Source: CAD feature listing. Evaluate the final solid. Frame: model axes, mm. A direction names the side the tool comes from. Give positions to 0.01 mm unless a question says otherwise; leave off trailing zeros. Order: outer loops, then holes, each group sorted by start corner. A loop starts at its lowest first (then second) coordinate and runs counter-clockwise, first axis right, second up. Notation, with made-up numbers: (3.25, -7) - (43.25, -7) arc R35 cw to (43.25, 29) - close; hole circle Ø9 at (54, -30). An arc over 180 degrees is marked (long way). Write each question's results on one line, items separated by ' | '. Start each with the question number.
Item 1: Line query: line 1 along Y through (x, z) = (0, 20); line 2 along X through (y, z) = (-5.5, 19); line 3 along Y through (x, z) = (2.5, 26). Output: solid intervals per line, ascending.
Item 2: Set-up query: faces 4 (the cylindrical face through (-0.04, -23.31, 21.84)), 5 (the flat face through (15, 15, 4)), 6 (the flat face through (2.5, -19, 20)), 7 (the flat face through (0, -19, 15)), 8 (the cylindrical face through (23.773, 23.602, 38.028)). Return all of +Z, -Z, +X, -X, +Y, -Y with unobstructed straight access to the full face (end or side cutting, diameter ignored); none if empty.
Item 3: Section D-D on z = 34. Output: boundary loops of the cut face in (x, y).
Item 4: Contact query for flat-ended pins moving along their axis: pin 1 Ø1 at (x, y) = (1.5, -16) entering from +Z; pin 2 Ø2 at (x, z) = (6, 19.5) entering from -Y; pin 3 Ø5 at (y, z) = (-24.5, 19) entering from -X. Output: stop coordinate, or through.
Item 5: Section C-C on x = 14.5. Output: boundary loops of the cut face in (y, z).
Item 6: Mould query, pull axis Z, two halves, no side actions, for faces 1 (the flat face through (0, -19, 25)), 2 (the flat face through (15, 15, 36)), 3 (the flat face through (-2.5, -19, 20)). Classes: released by +Z, released by -Z, zero draft, split by the parting line, or undercut.
Item 7: Section A-A on z = 20. Output: boundary loops of the cut face in (x, y), and give its area (3 significant figures).
Item 8: Section B-B on y = -1. Output: boundary loops of the cut face in (x, z).
```python
from build123d import *

# Parameters (mm, degrees)
EXTRUDE_1_DEPTH      = 40
SKETCH_1_4_R         = 3
EXTRUDE_3_DEPTH      = 4
EXTRUDE_4_DEPTH      = 2.5
EXTRUDE_4_DEPTH_BACK = 2.5
SKETCH_2_R           = 2.5


with BuildPart() as part:
    # Sketch 1 → Extrude 1 (new body)
    with BuildSketch(Plane.XY):
        with BuildLine():
            ThreePointArc((7.494638572, -0.283536021), (-5.303300859, -5.303300859), (-0.283536021, 7.494638572))
            Line((-0.283536021, 7.494638572), (4.048166637, 11.82634123))
            ThreePointArc((4.048166637, 11.82634123), (-10.169859462, -7.268009254), (12.5, 0))
            ThreePointArc((12.5, 0), (12.330435219, 2.05191796), (11.82634123, 4.048166637))
            Line((11.82634123, 4.048166637), (7.494638572, -0.283536021))
        make_face()
        with BuildLine():
            Line((4.048166637, 11.82634123), (-0.283536021, 7.494638572))
            ThreePointArc((-0.283536021, 7.494638572), (5.202089957, 5.40261604), (7.5, 0))
            ThreePointArc((7.5, 0), (7.498659523, -0.141793353), (7.494638572, -0.283536021))
            Line((7.494638572, -0.283536021), (11.82634123, 4.048166637))
            ThreePointArc((11.82634123, 4.048166637), (8.838834765, 8.838834765), (4.048166637, 11.82634123))
        make_face()
    extrude(amount=EXTRUDE_1_DEPTH)

    # Sketch 1_4 → Extrude 3 (add)
    with BuildSketch(Plane.XY):
        with BuildLine():
            Line((15.909902577, 23.68807717), (4.048166637, 11.82634123))
            ThreePointArc((4.048166637, 11.82634123), (8.838834765, 8.838834765), (11.82634123, 4.048166637))
            Line((11.82634123, 4.048166637), (23.68807717, 15.909902577))
            ThreePointArc((23.68807717, 15.909902577), (23.68807717, 23.68807717), (15.909902577, 23.68807717))
        make_face()
        with Locations((19.798989873, 19.798989873)):
            Circle(SKETCH_1_4_R, mode=Mode.SUBTRACT)
    extrude_3 = extrude(amount=EXTRUDE_3_DEPTH)

    # Mirror 1: Extrude 3 across plane
    add(extrude_3.mirror(Plane.XY.offset(20)))

    # Sketch 2 → Extrude 4 (add, two sides: drawn at the far end of the back side and taken through both)
    with BuildSketch(Plane(origin=(0, 0, 0), x_dir=(0, 0, -1), z_dir=(1, 0, 0)).offset(-EXTRUDE_4_DEPTH_BACK)):
        with BuildLine():
            Line((-25, -12.5), (-25, -25))
            ThreePointArc((-25, -25), (-20, -30), (-15, -25))
            Line((-15, -25), (-15, -12.5))
            ThreePointArc((-15, -12.5), (-15.105468435, -11.478451782), (-15.417424305, -10.5))
            Line((-15.417424305, -10.5), (-24.582575695, -10.5))
            ThreePointArc((-24.582575695, -10.5), (-24.894531565, -11.478451782), (-25, -12.5))
        make_face()
        with Locations((-20, -25)):
            Circle(SKETCH_2_R, mode=Mode.SUBTRACT)
    extrude(amount=EXTRUDE_4_DEPTH + EXTRUDE_4_DEPTH_BACK)


solid = part.part
```
Evaluation:
1) line 1: y = -30 to -27.5, -22.5 to -7.5, 7.5 to 12.5 | line 2: x = -11.22 to -5.1, 5.1 to 11.22 | line 3: y = -12.25 to -7.07, 7.07 to 12.25
2) face 4: +X, -X | face 5: +X, +Y | face 6: +Z, -Z, +X, -Y | face 7: -Z, +X, -X, -Y | face 8: +Z, -Z
3) outline: circle Ø25 at (0, 0); hole (7.49, -0.28) arc R7.5 ccw to (7.5, 0) arc R7.5 ccw (long way) to start
4) pin 1: stops at z = 25 | pin 2: stops at y = -11.46 | pin 3: stops at x = -2.5
5) outline: (6.72, 0) - (22.28, 0) - (22.28, 4) - (6.72, 4) - close; (6.72, 36) - (22.28, 36) - (22.28, 40) - (6.72, 40) - close
6) face 1: released by +Z | face 2: undercut | face 3: zero draft
7) outline: (-2.5, -30) - (2.5, -30) - (2.5, -27.5) - (-2.5, -27.5) - close; (-2.5, -22.5) - (2.5, -22.5) - (2.5, -12.25) arc R12.5 ccw (long way) to (-2.5, -12.25) - close; hole (7.49, -0.28) arc R7.5 ccw to (7.5, 0) arc R7.5 ccw (long way) to start | area: 377 mm^2
8) outline: (-12.46, 0) - (-7.43, 0) - (-7.43, 40) - (-12.46, 40) - close; (7.43, 0) - (12.46, 0) - (12.46, 40) - (7.43, 40) - close
